Read the model definition and answer for the solid it produces. Units are mm, in the model's axes. Give positions to 0.01 mm unless a question says otherwise; leave off trailing zeros. Loops run counter-clockwise (first coordinate to the right, second up) from the corner with the lowest first, then second, coordinate; pieces in that order, holes last. Notation, with made-up numbers: (-12.5, 83.5) - (-2.5, 83.5) arc R24 cw to (-2.5, 103.5) - close; hole circle Ø5 at (-14.75, 80.5). An arc over 180 degrees is marked (long way). Use a Markdown table: item, result. Add a question column.
Item 1: A cutting plane is placed at A-A (x = 0). Determine the outline of the cut face in (y, z).
Item 2: A cutting plane is placed at D-D (x = -63.5). Determine the outline of the cut face in (y, z).
Item 3: A cutting plane is placed at C-C (y = 9.75). Give the number of separate pieces and of enclosed holes in the cut face, plus the area to 3 significant figures.
Item 4: Each of these flat-tipped pins is pushed along its axis until it touches: P1, Ø1.5, axis at y = 7, z = -44.5, coming from the -X side; P2, Ø5, axis at x = 64, y = 3.5, coming from the -Z side; P3, Ø7, axis at x = 83.5, y = 7.5, coming from the +Z side. Where does it stop, or does it pass through?
Item 5: Consider probe 1 along X at (y, z) = (11.25, -1); probe 2 along X at (y, z) = (5.25, 46); probe 3 along Z at (x, y) = (44, 1.25). Determine where each line is inside the solid, lowest interval first. Write a range as [from, to].
Item 6: A cutting plane is placed at B-B (z = -63.5). Determine the outline of the cut face in (x, y).
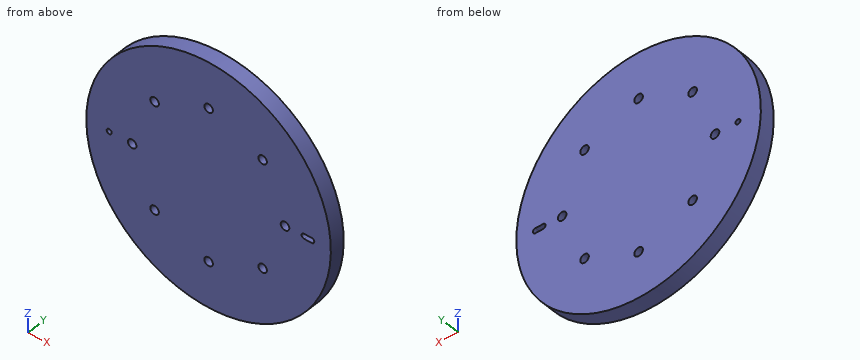
from build123d import *

# Parameters (mm, degrees)
SKETCH1_W               = 101.6
SKETCH1_H               = 12.7
CUT_EXTRUDE1_DEPTH      = 145.244271983
CUT_EXTRUDE1_DEPTH_BACK = 145.244271983
SKETCH2_R               = 3.5687
SKETCH3_R               = 2.0955
CUT_EXTRUDE4_DEPTH      = 31.75


with BuildPart() as part:
    # Sketch1 → Revolve1 (revolve)
    with BuildSketch(Plane(origin=(0, 0, 0), x_dir=(0, 0, -1), z_dir=(1, 0, 0)), mode=Mode.PRIVATE) as revolve1_sk:
        with Locations((50.8, 6.35)):
            Rectangle(SKETCH1_W, SKETCH1_H)
    revolve(revolve1_sk.sketch.rotate(Axis((0, 46.9, 0), (0, -1, 0)), 180), axis=Axis((0, 46.9, 0), (0, -1, 0)))

    # Sketch2 → Cut-Extrude1 (cut, two sides: drawn at the far end of the back side and taken through both)
    with BuildSketch(Plane(origin=(0, 12.7, 0), x_dir=(1, 0, 0), z_dir=(0, 1, 0)).offset(-CUT_EXTRUDE1_DEPTH_BACK)):
        with Locations(Location((0, 63.5, 0), (0, 0, 270))):
            Circle(SKETCH2_R)
        with Locations(Location((44.901280605, 44.901280605, 0), (0, 0, 270))):
            Circle(SKETCH2_R)
        with Locations(Location((63.5, 0, 0), (0, 0, 270))):
            Circle(SKETCH2_R)
        with Locations(Location((44.901280605, -44.901280605, 0), (0, 0, 270))):
            Circle(SKETCH2_R)
        with Locations(Location((0, -63.5, 0), (0, 0, 270))):
            Circle(SKETCH2_R)
        with Locations(Location((-44.901280605, -44.901280605, 0), (0, 0, 270))):
            Circle(SKETCH2_R)
        with Locations(Location((-63.5, 0, 0), (0, 0, 270))):
            Circle(SKETCH2_R)
        with Locations(Location((-44.901280605, 44.901280605, 0), (0, 0, 270))):
            Circle(SKETCH2_R)
    extrude(amount=CUT_EXTRUDE1_DEPTH + CUT_EXTRUDE1_DEPTH_BACK, mode=Mode.SUBTRACT)

    # Sketch3 → Cut-Extrude4 (cut)
    with BuildSketch(Plane(origin=(0, 12.7, 0), x_dir=(1, 0, 0), z_dir=(0, 1, 0))):
        with Locations(Location((-82.55, 0, 0), (0, 0, 270))):
            Circle(SKETCH3_R)
        with BuildLine():
            Line((79.375, -2.0955), (85.725, -2.0955))
            ThreePointArc((85.725, -2.0955), (87.8205, 0), (85.725, 2.0955))
            Line((85.725, 2.0955), (79.375, 2.0955))
            ThreePointArc((79.375, 2.0955), (77.2795, 0), (79.375, -2.0955))
        make_face()
    extrude(amount=-CUT_EXTRUDE4_DEPTH, mode=Mode.SUBTRACT)


solid = part.part
Geometry says:
| question | item | result |
|---|---|---|
| 1 | outline | (0, -101.6) - (12.7, -101.6) - (12.7, -67.07) - (0, -67.07) - close; (0, -59.93) - (12.7, -59.93) - (12.7, 59.93) - (0, 59.93) - close; (0, 67.07) - (12.7, 67.07) - (12.7, 101.6) - (0, 101.6) - close |
| 2 | outline | (0, -79.31) - (12.7, -79.31) - (12.7, -3.57) - (0, -3.57) - close; (0, 3.57) - (12.7, 3.57) - (12.7, 79.31) - (0, 79.31) - close |
| 3 | separate pieces | 1 |
| 3 | enclosed holes | 10 |
| 3 | area | 32,100 mm² |
| 4 | P1 | x = -91.7 |
| 4 | P2 | z = -80.87 |
| 4 | P3 | z = 62.63 |
| 5 | probe 1 | [-101.6, -84.39], [-80.71, -66.93], [-60.07, 60.07], [66.93, 77.53], [87.57, 101.6] |
| 5 | probe 2 | [-90.59, -48.3], [-41.51, 41.51], [48.3, 90.59] |
| 5 | probe 3 | [-91.58, -48.35], [-41.45, 41.45], [48.35, 91.58] |
| 6 | outline | (-79.31, 0) - (-3.57, 0) - (-3.57, 12.7) - (-79.31, 12.7) - close; (3.57, 0) - (79.31, 0) - (79.31, 12.7) - (3.57, 12.7) - close |
